```python
from build123d import *

# Parameters (mm, degrees)
SKETCH_1_R      = 1.5
EXTRUDE_1_DEPTH = 3
FILLET_1_R      = 3


with BuildPart() as part:
    # 草图1 → 凸台-拉伸1 (new body)
    with BuildSketch(Plane(origin=(0, 0, 0), x_dir=(1, 0, 0), z_dir=(0, 1, 0))):
        Polygon((0, 35), (0, 0), (42.142857143, 0), (42.142857143, 10), (10, 35), align=None)
        with Locations(Location((4, 7, 0), (0, 0, 270))):
            Circle(SKETCH_1_R, mode=Mode.SUBTRACT)
        with Locations(Location((15, 4, 0), (0, 0, 270))):
            Circle(SKETCH_1_R, mode=Mode.SUBTRACT)
        with Locations(Location((4, 15, 0), (0, 0, 270))):
            Circle(SKETCH_1_R, mode=Mode.SUBTRACT)
        with Locations(Location((35, 4, 0), (0, 0, 270))):
            Circle(SKETCH_1_R, mode=Mode.SUBTRACT)
        with Locations(Location((4, 23, 0), (0, 0, 270))):
            Circle(SKETCH_1_R, mode=Mode.SUBTRACT)
        with Locations(Location((4, 31, 0), (0, 0, 270))):
            Circle(SKETCH_1_R, mode=Mode.SUBTRACT)
    extrude(amount=EXTRUDE_1_DEPTH)

    # 圆角1
    fillet_1_edges = [part.edges().sort_by_distance(p)[0] for p in [
        (0, 1.5, 0),
        (0, 1.5, -35),
    ]]
    fillet(fillet_1_edges, radius=FILLET_1_R)


solid = part.part
```
Input: part model. Units: mm. Frame: model coordinates. Give positions to 0.01 mm unless a question says otherwise; leave off trailing zeros. Write each loop counter-clockwise with the first axis right and the second up, starting at its lowest first coordinate (ties: lowest second). Pieces come first, ordered by that corner, then holes. Notation, with made-up numbers: (-1.5, -10) - (39.5, -10) arc R7 ccw to (39.5, -1) - close; hole circle Ø11 at (70, 61.5). An arc over 180 degrees is marked (long way). Write item = value, one per line. Start each with the question number.
1. Section query A-A, the plane z = -4. Output: boundary loops of the cut face in (x, y), then the cut area to 3 significant figures.
2. First-contact query: pin 1 Ø1 at (y, z) = (1, -12.5) entering from +X. Flat tip, straight axial feed; report the tip coordinate or a pass-through.
3. Ray query, L1, parallel to X at y = 1.85, z = -4; L2, parallel to X at y = 1, z = -7; L3, parallel to Z at x = 3, y = 0.55. Return the intervals inside material, ascending.
4. Section query D-D, the plane x = 35. Output: boundary loops of the cut face in (y, z), then the cut area to 3 significant figures.
5. Mould query, pull axis Z, two halves, no side actions, for faces 1 (the cylindrical face through (3.1, 1.5, -32.2)), 2 (the flat face through (16, 0, -14)), 3 (the cylindrical face through (0.86, 1.52, -34.1)). Classes: released by +Z, released by -Z, zero draft, split by the parting line, or undercut.
6. Section query C-C, the plane x = 4. Output: boundary loops of the cut face in (y, z), then the cut area to 3 significant figures.
7. Section query B-B, the plane y = 2.05. Output: boundary loops of the cut face in (x, z).
Check sheet entries:
q1.outline = (0, 0) - (13.5, 0) - (13.5, 3) - (0, 3) - close; (16.5, 0) - (33.5, 0) - (33.5, 3) - (16.5, 3) - close; (36.5, 0) - (42.14, 0) - (42.14, 3) - (36.5, 3) - close
q1.area = 108 mm2
q2.pin_1 = 39.57
q3.L1 = 0 to 13.5, 16.5 to 33.5, 36.5 to 42.14
q3.L2 = 0 to 2.5, 5.5 to 42.14
q3.L3 = -35 to -32.12, -29.88 to -24.12, -21.88 to -16.12, -13.88 to -8.12, -5.88 to 0
q4.outline = (0, -15.56) - (3, -15.56) - (3, -5.5) - (0, -5.5) - close; (0, -2.5) - (3, -2.5) - (3, 0) - (0, 0) - close
q4.area = 37.7 mm2
q5.face_1 = undercut
q5.face_2 = zero draft
q5.face_3 = released by -Z
q6.outline = (0, -35) - (3, -35) - (3, -32.5) - (0, -32.5) - close; (0, -29.5) - (3, -29.5) - (3, -24.5) - (0, -24.5) - close; (0, -21.5) - (3, -21.5) - (3, -16.5) - (0, -16.5) - close; (0, -13.5) - (3, -13.5) - (3, -8.5) - (0, -8.5) - close; (0, -5.5) - (3, -5.5) - (3, 0) - (0, 0) - close
q6.area = 69.0 mm2
q7.outline = (0, -32) arc R3 ccw to (3, -35) - (10, -35) - (42.14, -10) - (42.14, 0) - (3, 0) arc R3 ccw to (0, -3) - close; hole circle Ø3 at (4, -31); hole circle Ø3 at (4, -23); hole circle Ø3 at (4, -15); hole circle Ø3 at (4, -7); hole circle Ø3 at (15, -4); hole circle Ø3 at (35, -4)
